```python
from build123d import *

# Parameters (mm, degrees)
F3_W     = 18
F3_H     = 15
F4_DEPTH = 80.001


with BuildPart() as f2:
    # F2: sweep along a path in F1
    with BuildLine(Plane.XY) as f2_path:
        CenterArc((0, 0), 28.500317, 0, 360)
    # F0 (on Front) → F2 (sweep)
    with BuildSketch(Plane.XZ):
        Polygon((68.741494, 0), (28.741494, 0), (28.741494, -80), (68.741494, -80), (68.741494, -70), (43.741494, -70), (43.741494, -60), (68.741494, -60), (68.741494, -50), (48.741494, -50), (48.741494, -30), (68.741494, -30), (68.741494, -20), (58.741494, -20), (58.741494, -10), (68.741494, -10), align=None)
    sweep(path=f2_path.line)

    # F3 (on Top) → F4 (cut, through all)
    with BuildSketch(Plane.XY):
        with Locations((0, 29.035522)):
            Rectangle(F3_W, F3_H)
    extrude(amount=-F4_DEPTH, mode=Mode.SUBTRACT)


solid = f2.part
```
Part model, mm, in its own coordinate system. A direction names the side the tool comes from. Coordinates: 2 decimals unless noted, no trailing zeros. Loops run counter-clockwise (first coordinate to the right, second up) from the corner with the lowest first, then second, coordinate; pieces in that order, holes last. Notation, with made-up numbers: (80, 31) - (86, 31) arc R20 ccw to (86, 70) - close; hole circle Ø4 at (49, 42). An arc over 180 degrees is marked (long way). Write item = value, one per line. Start each with the question number.
Item 1: Flat gauge pins, fed straight in: pin 1 Ø3 at (x, z) = (-12, -33) entering from -Y; pin 2 Ø3 at (x, z) = (-25.5, -34.5) entering from -Y; pin 3 Ø1.5 at (x, z) = (-34, -54) entering from +Y (3 decimals). Where does each tip first touch, or does it go through?
Item 2: Cut at B-B, the plane x = -52. State how many separate pieces and enclosed holes the cut face has, and give its area (3 significant figures).
Item 3: Cut at D-D, the plane z = -56. Give the cut face in (x, y).
Item 4: Wall check: L1, parallel to Z at x = -54, y = 4.5; L2, parallel to Z at x = 19, y = -63; L3, parallel to Y at x = 0, z = -28. Give the ranges that are in metal, low to high. Write a range as from..to.
Item 5: Mould opens along Y. For faces 3 (the flat face through (9, 32, -39)), 4 (the cylindrical face through (-1.14, -28.72, -40.56)), 5 (the cylindrical face through (41.72, 13.14, -64.93)) say: released by +Y, released by -Y, zero draft, split by the parting line, or undercut.
Item 6: Cut at A-A, the plane z = -44.5. Give the cut face in (x, y).
Item 7: 3-axis set-ups, long thin cutter, end or side, ignore diameter. For faces 1 (the cylindrical face through (45.025, -18.668, -39.86)), 2 (the flat face through (0, 36.536, -39)): which of +Z, -Z, +X, -X, +Y, -Y reach the whole face in a straight line?
The answers:
q1.pin_1 = -47.6
q1.pin_2 = -42.42
q1.pin_3 = 60.165
q2.separate_pieces = 3
q2.enclosed_holes = 0
q2.area = 4,140 mm2
q3.outline = circle Ø137.48 at (0, 0); hole (-9, 27.3) arc R28.74 ccw (long way) to (9, 27.3) - (9, 36.54) - (-9, 36.54) - close
q4.L1 = -80..-70, -60..-50, -30..0
q4.L2 = -80..-70, -60..-50, -30..-20, -10..0
q4.L3 = -68.74..-28.74, 36.54..68.74
q5.face_3 = undercut
q5.face_4 = undercut
q5.face_5 = split by the parting line
q6.outline = circle Ø97.48 at (0, 0); hole (-9, 27.3) arc R28.74 ccw (long way) to (9, 27.3) - (9, 36.54) - (-9, 36.54) - close
q7.face_1 = none
q7.face_2 = +Z, -Z
